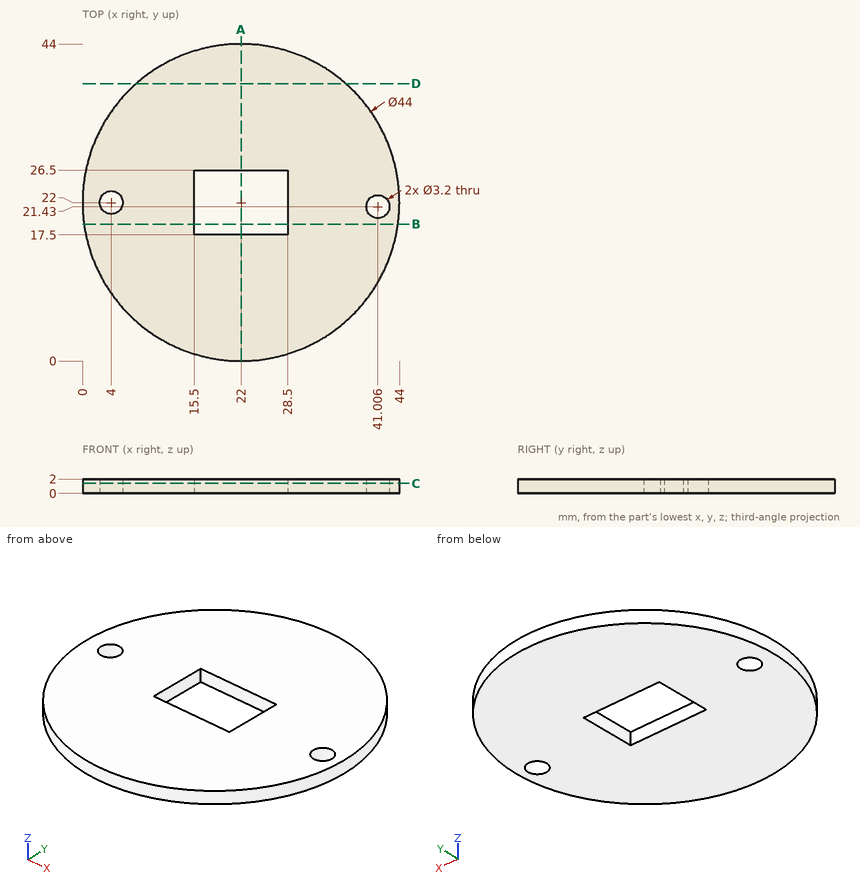
Study the drawing (mm; zero at the part's minimum x, y, z) and answer. Give positions to 0.01 mm unless a question says otherwise; leave off trailing zeros. Order: outer loops, then holes, each group sorted by start corner. A loop starts at its lowest first (then second) coordinate and runs counter-clockwise, first axis right, second up.
1. Section D-D, the plane y = 38.5 is taken. Determine the outline of the cut face in (x, z).
Result sheet:
outline: (7.45, 0) - (36.55, 0) - (36.55, 2) - (7.45, 2) - close
2. Section B-B, the plane y = 19 is taken. Determine the outline of the cut face in (x, z) (1 decimal).
Result sheet:
outline: (0.2, 0) - (15.5, 0) - (15.5, 2) - (0.2, 2) - close; (28.5, 0) - (43.8, 0) - (43.8, 2) - (28.5, 2) - close
3. Straight lines are drawn through the part: L1, parallel to Y at x = 22, z = 0.1; L2, parallel to Y at x = 4, z = 1.8; L3, parallel to X at y = 7.5, z = 1.1 (1 decimal). For each, find the intervals that lie inside material, in ascending order.
Result sheet:
L1: y = 0 to 17.5, 26.5 to 44
L2: y = 9.35 to 20.4, 23.6 to 34.65
L3: x = 5.5 to 38.5
4. Section C-C, the plane z = 1.4 is taken. Determine the outline of the cut face in (x, y).
Result sheet:
outline: circle Ø44 at (22, 22); hole circle Ø3.2 at (4, 22); hole (15.5, 17.5) - (28.5, 17.5) - (28.5, 26.5) - (15.5, 26.5) - close; hole circle Ø3.2 at (41.01, 21.43)
5. Section A-A, the plane x = 22 is taken. Determine the outline of the cut face in (y, z).
Result sheet:
outline: (0, 0) - (17.5, 0) - (17.5, 2) - (0, 2) - close; (26.5, 0) - (44, 0) - (44, 2) - (26.5, 2) - close
6. Each of these flat-tipped pins is pushed along its axis until it touches: P1, Ø1, axis at x = 22, z = 1, coming from the -Y side; P2, Ø1, axis at y = 20, z = 0.5, coming from the -X side; P3, Ø1.9, axis at x = 41.01, y = 21.43, coming from the +Z side; P4, Ø1, axis at x = 4.5, z = 1, coming from the +Y side (1 decimal). Where does it stop, or does it pass through?
Result sheet:
P1: stops at y = 0
P2: stops at x = 0.05
P3: passes through
P4: stops at y = 36
